```python
from build123d import *

# Parameters (mm, degrees)
F1_DEPTH = 0.3


with BuildPart() as f1:
    # F0 (on Top) → F1 (new body)
    with BuildSketch(Plane.XY):
        Polygon((100, 48.856538), (-90, 48.856538), (-90, 48.456538), (99.6, 48.456538), (99.6, 28.856538), (-90, 28.856538), (-90, 28.456538), (-90, 8.856538), (-90, 8.456538), (99.6, 8.456538), (99.6, -11.143462), (-90, -11.143462), (-90, -11.543462), (-90, -31.143462), (-90, -31.543462), (99.6, -31.543462), (99.6, -51.143462), (-90, -51.143462), (-90, -51.543462), (-90, -71.143462), (-90, -71.543462), (99.6, -71.543462), (99.6, -91.143462), (-90, -91.143462), (-90, -91.543462), (-90, -111.143462), (-89.6, -111.143462), (-89.6, -91.543462), (100, -91.543462), (100, -71.543462), (100, -71.143462), (-89.6, -71.143462), (-89.6, -51.543462), (100, -51.543462), (100, -31.543462), (100, -31.143462), (-89.6, -31.143462), (-89.6, -11.543462), (100, -11.543462), (100, 8.456538), (100, 8.856538), (-89.6, 8.856538), (-89.6, 28.456538), (100, 28.456538), (100, 48.456538), align=None)
        Polygon((100, -111.143462), (-89.6, -111.143462), (-90, -111.143462), (-90, -111.543462), (99.6, -111.543462), (99.6, -131.143462), (-90, -131.143462), (-90, -131.543462), (-89.6, -131.543462), (100, -131.543462), (100, -111.543462), align=None)
    extrude(amount=F1_DEPTH)


solid = f1.part
```
Part model, mm, in its own coordinate system. Round coordinates to 2 decimals unless told otherwise and drop trailing zeros. Write each loop counter-clockwise with the first axis right and the second up, starting at its lowest first coordinate (ties: lowest second). Pieces come first, ordered by that corner, then holes. Notation, with made-up numbers: M -27,40 L 11,40 A28 ccw 11,71 Z; hole C 82.5,42.5 d10. An arc over 180 degrees is marked long. One line per question, with ' | ' between items.
(1) Pin check, flat tip, straight feed: pin 1 (1.5 mm diameter, centred on x = 65.5, y = -13.5, fed in from +Z). Stop position of the tip, or through.
Answer key:
pin 1: passes through
(2) Saw through at A-A on x = 69. Count the separate pieces of the cut face and the enclosed holes in it, then the cut area to 3 significant figures.
Answer key:
separate pieces: 10 | enclosed holes: 0 | area: 1.20 mm^2
(3) Probe line 1 along X through (y, z) = (-43.5, 0.25); line 2 along X through (y, z) = (26.5, 0.2). List the from-to ranges inside material, lowest first.
Answer key:
line 1: x = 99.6 to 100 | line 2: x = -90 to -89.6
(4) Saw through at B-B on y = -15. Write the cut outline in (x, z), then the cut area to 3 significant figures.
Answer key:
outline: M -90,0 L -89.6,0 L -89.6,0.3 L -90,0.3 Z | area: 0.120 mm^2
